Source: CAD feature listing. Evaluate the final solid. Frame: model axes, mm. A direction names the side the tool comes from. Round coordinates to 2 decimals unless told otherwise and drop trailing zeros. Order: outer loops, then holes, each group sorted by start corner. A loop starts at its lowest first (then second) coordinate and runs counter-clockwise, first axis right, second up. Notation, with made-up numbers: (-9, 70) - (19, 70) arc R30 cw to (19, 100) - close; hole circle Ø8 at (77, 69). An arc over 180 degrees is marked (long way). Return JSON: item names as keys, results as strings. Group by question number.
1) Contact query for flat-ended pins moving along their axis: P1, Ø20, axis at x = -36, z = -37.5, coming from the -Y side; P2, Ø8, axis at x = 19.5, z = -62, coming from the +Y side; P3, Ø3, axis at y = 2.5, z = -38, coming from the -X side; P4, Ø5.5, axis at y = 10, z = -63.5, coming from the -X side. Output: stop coordinate, or through.
2) Mould query, pull axis Z, two halves, no side actions, for faces 4 (the flat face through (28, 11, -75)), 5 (the cylindrical face through (-25.508, 50.675, -40.804)), 6 (the flat face through (-44.04, 38, -29.75)). Classes: pulls with the +Z half, pulls with the -Z half, needs draft (parallel to the pull), parting line crosses it, or undercut.
3) Ray query, line 1 (Z direction, x = 28, y = 9); line 2 (Z direction, x = -36, y = 50); line 3 (X direction, y = 13, z = -60). Return the intervals inside material, ascending. Write a range as from..to.
4) Section C-C, the plane x = -36. Return loops of the section in (y, z), plus the area to 3 significant figures.
5) Section D-D, the plane y = 57.5. Return loops of the section in (x, z), plus the area to 3 significant figures.
6) Access query for faces 1 (the flat face through (0, 9, -59)), 2 (the flat face through (21, 18, -59)), 3 (the flat face through (21, 18, -16)). Directions: +Z, -Z, +X, -X, +Y, -Y. A direction counts if a zero-diameter tool reaches every point of the face in a straight line with its end or side. Return the directions, or none.
7) Section B-B, the plane z = -15. Return loops of the section in (x, y).
8) Section A-A, the plane x = 28. Return loops of the section in (y, z), plus the area to 3 significant figures.
```python
from build123d import *

# Parameters (mm, degrees)
SKETCH2_W            = 56
SKETCH2_H            = 75
BOSS_EXTRUDE1_DEPTH  = 18
SKETCH3_W            = 32
SKETCH3_H            = 75
CUT_EXTRUDE1_DEPTH   = 6
SKETCH6_R            = 6
CUT_EXTRUDE2_DEPTH   = 47
SKETCH7_W            = 56
SKETCH7_H            = 12
BOSS_EXTRUDE2_DEPTH  = 45
CUT_EXTRUDE3_DEPTH   = 45
SKETCH9_W            = 36
SKETCH9_H            = 25
BOSS_EXTRUDE5_DEPTH  = 12
SKETCH10_R           = 18
BOSS_EXTRUDE9_DEPTH  = 25
SKETCH11_R           = 11
CUT_EXTRUDE4_DEPTH   = 25
BOSS_EXTRUDE10_DEPTH = 12


with BuildPart() as part:
    # Sketch2 → Boss-Extrude1 (new body)
    with BuildSketch(Plane(origin=(0, 0, 0), x_dir=(1, 0, 0), z_dir=(0, 1, 0))):
        with Locations((28, 37.5)):
            Rectangle(SKETCH2_W, SKETCH2_H)
    extrude(amount=BOSS_EXTRUDE1_DEPTH)

    # Sketch3 → Cut-Extrude1 (cut)
    with BuildSketch(Plane.XZ):
        with Locations((28, -37.5)):
            Rectangle(SKETCH3_W, SKETCH3_H)
    extrude(amount=-CUT_EXTRUDE1_DEPTH, mode=Mode.SUBTRACT)

    # Sketch6 → Cut-Extrude2 (cut)
    with BuildSketch(Plane(origin=(0, 18, 0), x_dir=(1, 0, 0), z_dir=(0, 1, 0))):
        with Locations((28, 15)):
            Circle(SKETCH6_R)
        with Locations((28, 60)):
            Circle(SKETCH6_R)
    extrude(amount=-CUT_EXTRUDE2_DEPTH, mode=Mode.SUBTRACT)

    # Sketch7 → Boss-Extrude2 (add)
    with BuildSketch(Plane(origin=(0, 18, 0), x_dir=(1, 0, 0), z_dir=(0, 1, 0))):
        with Locations((28, 37.5)):
            Rectangle(SKETCH7_W, SKETCH7_H)
    extrude(amount=BOSS_EXTRUDE2_DEPTH)

    # Sketch8 → Cut-Extrude3 (cut)
    with BuildSketch(Plane(origin=(0, 0, -43.5), x_dir=(-1, 0, 0), z_dir=(0, 0, -1))):
        Polygon((-56, 18), (0, 63), (-56, 63), align=None)
    extrude(amount=-CUT_EXTRUDE3_DEPTH, mode=Mode.SUBTRACT)

    # Sketch9 → Boss-Extrude5 (add)
    with BuildSketch(Plane(origin=(0, 0, -43.5), x_dir=(-1, 0, 0), z_dir=(0, 0, -1))):
        with Locations((18, 50.5)):
            Rectangle(SKETCH9_W, SKETCH9_H)
    extrude(amount=-BOSS_EXTRUDE5_DEPTH)

    # Sketch10 → Boss-Extrude9 (add)
    with BuildSketch(Plane(origin=(0, 63, 0), x_dir=(1, 0, 0), z_dir=(0, 1, 0))):
        with Locations((-36, 37.5)):
            Circle(SKETCH10_R)
    extrude(amount=-BOSS_EXTRUDE9_DEPTH)

    # Sketch11 → Cut-Extrude4 (cut)
    with BuildSketch(Plane(origin=(0, 63, 0), x_dir=(1, 0, 0), z_dir=(0, 1, 0))):
        with Locations((-36, 37.5)):
            Circle(SKETCH11_R)
    extrude(amount=-CUT_EXTRUDE4_DEPTH, mode=Mode.SUBTRACT)

    # Sketch12 → Boss-Extrude10 (add)
    with BuildSketch(Plane(origin=(0, 0, -43.5), x_dir=(-1, 0, 0), z_dir=(0, 0, -1))):
        Polygon((19.029437252, 38), (0, 0), (0, 38), align=None)
    extrude(amount=-BOSS_EXTRUDE10_DEPTH)


solid = part.part
```
Geometry check:
{
 "1": {"P1": "through", "P2": "y = 18", "P3": "x = -2", "P4": "x = 0"},
 "2": {"face 4": "pulls with the -Z half", "face 5": "undercut", "face 6": "needs draft"},
 "3": {"line 1": "-75..-66, -54..-21, -9..0", "line 2": "-55.5..-48.5, -26.5..-19.5", "line 3": "0..22, 34..56"},
 "4": {"outline": "(38, -55.5) - (63, -55.5) - (63, -48.5) - (38, -48.5) - close; (38, -26.5) - (63, -26.5) - (63, -19.5) - (38, -19.5) - close", "area": "350 mm2"},
 "5": {"outline": "(-19.03, -43.5) - (6.84, -43.5) - (6.84, -31.5) - (-19.03, -31.5) arc R18 ccw (long way) to start; hole circle Ø22 at (-36, -37.5)", "area": "940 mm2"},
 "6": {"face 1": "-Z, -X, +Y, -Y", "face 2": "-Z, +X, -X, +Y", "face 3": "+Z, +X, -X, +Y"},
 "7": {"outline": "(0, 0) - (12, 0) - (12, 6) - (22, 6) - (22, 18) - (0, 18) - close; (34, 6) - (44, 6) - (44, 0) - (56, 0) - (56, 18) - (34, 18) - close"},
 "8": {"outline": "(6, -75) - (18, -75) - (18, -66) - (6, -66) - close; (6, -54) - (18, -54) - (18, -43.5) - (40.5, -43.5) - (40.5, -31.5) - (18, -31.5) - (18, -21) - (6, -21) - close; (6, -9) - (18, -9) - (18, 0) - (6, 0) - close", "area": "882 mm2"}
}
